Source: CAD feature listing. Evaluate the final solid. Frame: model axes, mm. A direction names the side the tool comes from. Give positions to 0.01 mm unless a question says otherwise; leave off trailing zeros. Order: outer loops, then holes, each group sorted by start corner. A loop starts at its lowest first (then second) coordinate and runs counter-clockwise, first axis right, second up. Notation, with made-up numbers: M 23,33 L 76,33 A9 cw 76,48 Z; hole C -20.5,-38.75 d9. An arc over 180 degrees is marked long. Return JSON: item names as keys, results as strings.
from build123d import *

# Parameters (mm, degrees)
F1_DEPTH = 25.4
F2_W     = 38.1
F2_H     = 12.7
F3_DEPTH = 50.8
F4_W     = 25.4
F4_H     = 25.4
F5_DEPTH = 38.1
F6_R     = 3.175


with BuildPart() as f1:
    # F0 (on Front) → F1 (new body)
    with BuildSketch(Plane.XZ):
        with BuildLine():
            ThreePointArc((0, 25.4), (25.4, 0), (0, -25.4))
            Line((0, -25.4), (-139.7, -25.4))
            Line((-139.7, -25.4), (-139.7, -28.575))
            Line((-139.7, -28.575), (0, -28.575))
            ThreePointArc((0, -28.575), (28.575, 0), (0, 28.575))
            Line((0, 28.575), (-139.7, 28.575))
            Line((-139.7, 28.575), (-139.7, 25.4))
            Line((-139.7, 25.4), (0, 25.4))
        make_face()
    extrude(amount=F1_DEPTH)

    # F2 (on face) → F3 (join)
    with BuildSketch(Plane(origin=(-139.7, 0, 0), x_dir=(0, -1, 0), z_dir=(-1, 0, 0))):
        with Locations((12.7, 19.05)):
            Rectangle(F2_W, F2_H)
        with Locations((12.7, -19.05)):
            Rectangle(F2_W, F2_H)
    extrude(amount=-F3_DEPTH)

    # F4 (on face) → F5 (join)
    with BuildSketch(Plane(origin=(0, 0, -28.575), x_dir=(1, 0, 0), z_dir=(0, 0, -1))):
        with Locations((-25.4, 12.7)):
            Rectangle(F4_W, F4_H)
    extrude(amount=F5_DEPTH)

    # F6
    f6_edges = [f1.edges().sort_by_distance(p)[0] for p in [
        (-38.1, -25.4, -47.625),
        (-38.1, 0, -47.625),
        (-12.7, -25.4, -47.625),
        (-12.7, 0, -47.625),
    ]]
    fillet(f6_edges, radius=F6_R)


solid = f1.part
1. Section query C-C (y = -6). Return loops of the section in (x, z) (3 decimals), then the cut area to 3 significant figures.
Evaluation:
{"outline": "M -139.7,-28.575 L -38.1,-28.575 L -38.1,-66.675 L -12.7,-66.675 L -12.7,-28.575 L 0,-28.575 A28.575 ccw 0,28.575 L -139.7,28.575 L -139.7,12.7 L -88.9,12.7 L -88.9,25.4 L 0,25.4 A25.4 cw 0,-25.4 L -88.9,-25.4 L -88.9,-12.7 L -139.7,-12.7 Z", "area": "3,410 mm^2"}
2. Section query D-D (x = -100). Return loops of the section in (y, z) (3 decimals).
Evaluation:
{"outline": "M -31.75,-25.4 L -25.4,-25.4 L -25.4,-28.575 L 0,-28.575 L 0,-25.4 L 6.35,-25.4 L 6.35,-12.7 L -31.75,-12.7 Z; M -31.75,12.7 L 6.35,12.7 L 6.35,25.4 L 0,25.4 L 0,28.575 L -25.4,28.575 L -25.4,25.4 L -31.75,25.4 Z"}
3. Draft query along Z for faces 1 (the face through (-115, 3, 25.4)), 2 (the face through (-38.1, -13, -47)), 3 (the face through (-88.9, -12, -19)), 4 (the face through (25.394, -12.522, 0.559)). Return one class per face: pulls with the +Z half, pulls with the -Z half, needs draft (parallel to the pull), parting line crosses it, or undercut.
Evaluation:
{"face 1": "pulls with the +Z half", "face 2": "needs draft", "face 3": "undercut", "face 4": "undercut"}
4. Set-up query: faces 5 (the face through (-115, 3, -25.4)), 6 (the face through (-115, -12, -12.7)), 7 (the face through (-115, -29, -25.4)). Return all of +Z, -Z, +X, -X, +Y, -Y with unobstructed straight access to the full face (end or side cutting, diameter ignored); none if empty.
Evaluation:
{"face 5": "-Z, +X, -X, +Y", "face 6": "-X, +Y, -Y", "face 7": "-Z, +X, -X, -Y"}
5. Section query A-A (x = -78.5). Return loops of the section in (y, z) (3 decimals), then the cut area to 3 significant figures.
Evaluation:
{"outline": "M -25.4,-28.575 L 0,-28.575 L 0,-25.4 L -25.4,-25.4 Z; M -25.4,25.4 L 0,25.4 L 0,28.575 L -25.4,28.575 Z", "area": "161 mm^2"}
6. Section query B-B (z = -38.5). Return loops of the section in (x, y) (3 decimals), then the cut area to 3 significant figures.
Evaluation:
{"outline": "M -38.1,-22.225 A3.175 ccw -34.925,-25.4 L -15.875,-25.4 A3.175 ccw -12.7,-22.225 L -12.7,-3.175 A3.175 ccw -15.875,0 L -34.925,0 A3.175 ccw -38.1,-3.175 Z", "area": "637 mm^2"}
7. Ray query, probe 1 along Z at (x, y) = (-122, -18) (3 decimals); probe 2 along Z at (x, y) = (-79.5, -12.5) (3 decimals); probe 3 along X at (y, z) = (1, -24). Return the intervals inside material, ascending.
Evaluation:
{"probe 1": "z = -28.575 to -12.7, 12.7 to 28.575", "probe 2": "z = -28.575 to -25.4, 25.4 to 28.575", "probe 3": "x = -139.7 to -88.9"}
8. First-contact query: pin 1 (10 mm diameter, centred on y = -22, z = -53.5, fed in from +X); pin 2 (3 mm diameter, centred on x = -111.5, y = 3, fed in from -Z); pin 3 (7 mm diameter, centred on x = -108, y = -27.5, fed in from -Z) (3 decimals). Flat tips, straight axial feed; report the tip coordinate or a pass-through.
Evaluation:
{"pin 1": "stops at x = -12.7", "pin 2": "stops at z = -25.4", "pin 3": "stops at z = -28.575"}
